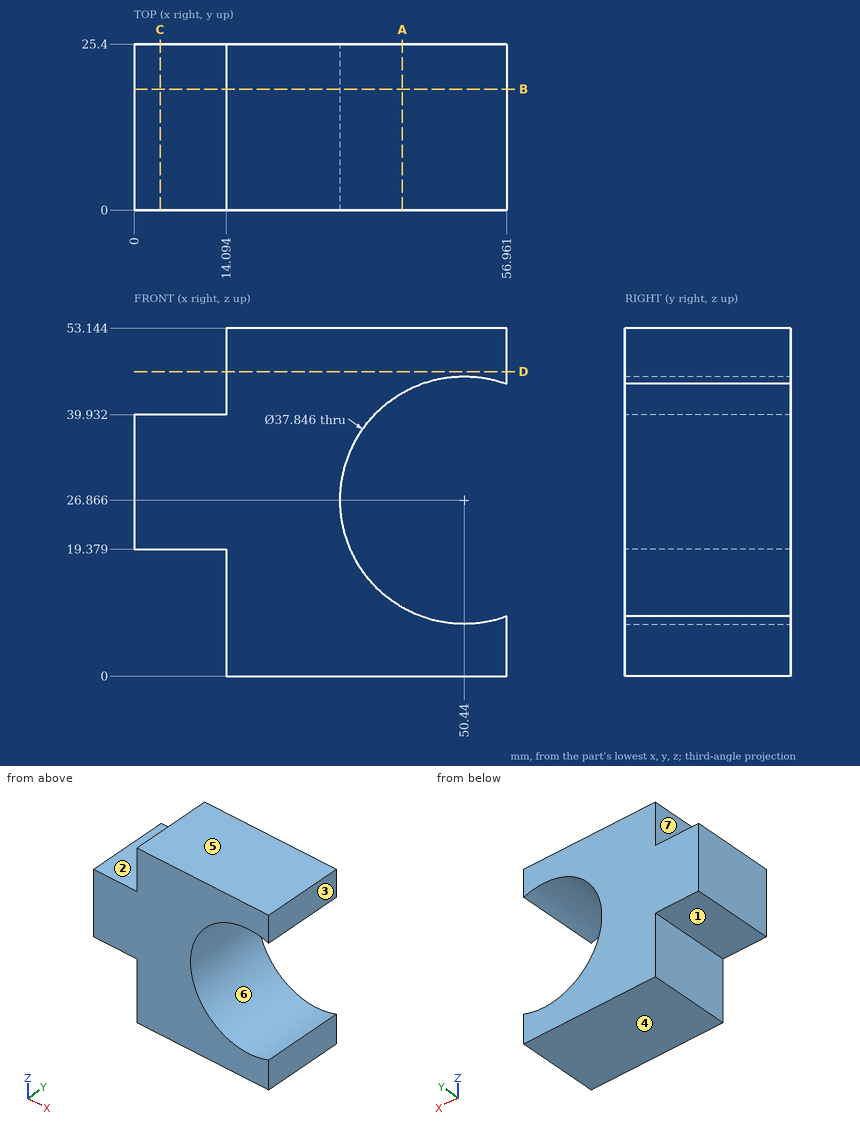
Verification items for this drawing (mm, ordinates from the low corner). A direction names the side the tool comes from. Give positions to 0.01 mm unless a question says otherwise; leave off trailing zeros. Loops run counter-clockwise (first coordinate to the right, second up) from the corner with the lowest first, then second, coordinate; pieces in that order, holes last. Notation, with made-up numbers: M 70,-23.75 L 92,-23.75 A19 ccw 92,4.25 Z; hole C -3,37 d9. An arc over 180 degrees is marked long. Answer as CSV lines item,"result".
Item 1: Depth check by flat-ended pin: P1, Ø2, axis at y = 20.5, z = 43.5, coming from the -X side; P2, Ø4, axis at x = 8.5, y = 14.5, coming from the +Z side. Enter the tip coordinate at first touch or a pass-through.
Values:
P1,"stops at x = 14.09"
P2,"stops at z = 39.93"
Item 2: Access from +Z, -Z, +X, -X, +Y, -Y to the whole of each face (thin tool, end or side, straight path). Record for the marked faces 1, 2 and 3.
Values:
face 1,"-Z, -X, +Y, -Y"
face 2,"+Z, -X, +Y, -Y"
face 3,"+Z, -Z, +X, +Y, -Y"
Item 3: Cross-section at B-B on y = 18.5. Record the cut outline in (x, z) (1 decimal).
Values:
outline,"M 0,19.4 L 14.1,19.4 L 14.1,0 L 57,0 L 57,9.1 A18.9 cw long 57,44.6 L 57,53.1 L 14.1,53.1 L 14.1,39.9 L 0,39.9 Z"
Item 4: Material ranges on line 1 (Z direction, x = 4, y = 23.25); line 2 (X direction, y = 16.25, z = 7.5); line 3 (Z direction, x = 34.5, y = 4.5) (1 decimal), recorded low to high.
Values:
line 1,"z = 19.38 to 39.93"
line 2,"x = 14.09 to 56.96"
line 3,"z = 0 to 16.7, 37.1 to 53.1"
Item 5: Cross-section at D-D on z = 46.5. Record the cut outline in (x, y).
Values:
outline,"M 14.09,0 L 56.96,0 L 56.96,25.4 L 14.09,25.4 Z"
Item 6: Cross-section at A-A on x = 41. Record the cut outline in (y, z) (1 decimal), and give its area (3 significant figures).
Values:
outline,"M 0,0 L 25.4,0 L 25.4,10.5 L 0,10.5 Z; M 0,43.3 L 25.4,43.3 L 25.4,53.1 L 0,53.1 Z"
area,"517 mm²"
Item 7: Cross-section at C-C on x = 4. Record the cut outline in (y, z), and give its area (3 significant figures).
Values:
outline,"M 0,19.38 L 25.4,19.38 L 25.4,39.93 L 0,39.93 Z"
area,"522 mm²"
Item 8: Release check for a two-part mould opening along Z. For the marked faces 4, 5, 6 and 7 record: pulls with the +Z half, pulls with the -Z half, needs draft (parallel to the pull), parting line crosses it, or undercut.
Values:
face 4,"pulls with the -Z half"
face 5,"pulls with the +Z half"
face 6,"undercut"
face 7,"needs draft"
